from build123d import *

# Parameters (mm, degrees)
F0_W           = 31.75
F0_H           = 31.75
F1_DEPTH       = 38.1
F3_D           = 5.1054
F3_CBORE_D     = 8.73125
F3_CBORE_DEPTH = 25.4
F5_DEPTH       = 31.751
F7_D           = 4.0386
F7_DEPTH       = 9.49325
F7_TIP         = 1.213317848


with BuildPart() as f1:
    # F0 (on Top) → F1 (new body)
    with BuildSketch(Plane.XY):
        Rectangle(F0_W, F0_H)
    extrude(amount=F1_DEPTH)

    # F3 (through all)
    with Locations(Plane(origin=(0, 0, 0), x_dir=(1, 0, 0), z_dir=(0, 0, -1))):
        with Locations((0, 0)):
            CounterBoreHole(F3_D / 2, F3_CBORE_D / 2, F3_CBORE_DEPTH)

    # F4 (on face) → F5 (cut, through all)
    with BuildSketch(Plane.XZ.offset(15.875)):
        Polygon((34.4816722517, 22.1809802753), (33.3208667558, 31.6349823697), (8.1101945041, 28.5395010472), (9.271, 19.0854989528), align=None)
    extrude(amount=-F5_DEPTH, mode=Mode.SUBTRACT)

    # F7
    with Locations(Plane.XY.offset(38.1)):
        with Locations((12.065, -9.525), (12.065, 9.525)):
            Hole(F7_D / 2, depth=F7_DEPTH)
            with Locations((0, 0, -(F7_DEPTH + F7_TIP / 2))):  # 118° drill point
                Cone(0, F7_D / 2, F7_TIP, mode=Mode.SUBTRACT)


solid = f1.part
The model under review builds one solid part; all positions refer to its coordinate system, in mm. A direction names the side the tool comes from. Round coordinates to 2 decimals unless told otherwise and drop trailing zeros. Write each loop counter-clockwise with the first axis right and the second up, starting at its lowest first coordinate (ties: lowest second). Pieces come first, ordered by that corner, then holes. Notation, with made-up numbers: M 39.5,68 L 86.5,68 A33 ccw 86.5,107 Z; hole C 21.5,29.5 d5. An arc over 180 degrees is marked long. Use a Markdown table: item, result. Add a question column.
Q1. Machinability: for faces 1 (the face through (12.527, -0.222, 19.485)), 2 (the face through (10.2, -10.3, 33.4)), 3 (the face through (-3.46, 2.66, 12.52)), which of the approach directions +Z, -Z, +X, -X, +Y, -Y give a long, thin tool a straight path to every point of the face, cutting with its end or side? Answer none if there is none.
Q2. The part is to be moulded in two halves that separate along Z. For faces 4 (the face through (8.682, -0.222, 23.879)), 5 (the face through (2, 2, 25.4)), 6 (the face through (0, 15.875, 19)), 7 (the face through (-4, 0, 38.1)), say which applies: pulls with the +Z half, pulls with the -Z half, needs draft (parallel to the pull), parting line crosses it, or undercut.
Q3. To check wall thickness, follow line 1 (Y direction, x = 0, z = 28) (3 decimals); line 2 (Z direction, x = 12.5, y = -2.5); line 3 (X direction, y = 1.5, z = 22.5) (3 decimals). State the ranges of each line that lie inside material, in increasing order.
Q4. Insertion check: pin 1 (4.5 mm diameter, centred on x = 0, y = 0, fed in from -Z); pin 2 (3 mm diameter, centred on y = 9.5, z = 24.5, fed in from +X); pin 3 (1 mm diameter, centred on y = -8.5, z = 27, fed in from +X); pin 4 (7 mm diameter, centred on x = 0, y = 0, fed in from -Z). Each pin has a flat end and moves straight along its axis. Give the tip position at first contact, or say it passes through.
Q5. We need section B-B, the plane x = 0. State the section outline as (y, z) points (3 decimals), plus the area to 3 significant figures.
Q6. We need section D-D, the plane z = 32.5. State the section outline as (x, y) points (3 decimals).
Q7. We need section C-C, the plane z = 4. State the section outline as (x, y) points (3 decimals).
Q8. We need section A-A, the plane y = 0. State the section outline as (x, z) points (1 decimal), plus the area to 3 significant figures.
Findings below:
| question | item | result |
|---|---|---|
| 1 | face 1 | +Y, -Y |
| 1 | face 2 | +Z |
| 1 | face 3 | -Z |
| 2 | face 4 | undercut |
| 2 | face 5 | pulls with the -Z half |
| 2 | face 6 | needs draft |
| 2 | face 7 | pulls with the +Z half |
| 3 | line 1 | y = -15.875 to -2.553, 2.553 to 15.875 |
| 3 | line 2 | z = 0 to 19.48, 29.08 to 38.1 |
| 3 | line 3 | x = -15.875 to -4.1, 4.1 to 8.852 |
| 4 | pin 1 | passes through |
| 4 | pin 2 | stops at x = 8.79 |
| 4 | pin 3 | stops at x = 8.36 |
| 4 | pin 4 | stops at z = 25.4 |
| 5 | outline | M -15.875,0 L -4.366,0 L -4.366,25.4 L -2.553,25.4 L -2.553,38.1 L -15.875,38.1 Z; M 2.553,25.4 L 4.366,25.4 L 4.366,0 L 15.875,0 L 15.875,38.1 L 2.553,38.1 Z |
| 5 | area | 923 mm² |
| 6 | outline | M -15.875,-15.875 L 15.875,-15.875 L 15.875,15.875 L -15.875,15.875 Z; hole C 0,0 d5.105; hole C 12.065,-9.525 d4.039; hole C 12.065,9.525 d4.039 |
| 7 | outline | M -15.875,-15.875 L 15.875,-15.875 L 15.875,15.875 L -15.875,15.875 Z; hole C 0,0 d8.731 |
| 8 | outline | M -15.9,0 L -4.4,0 L -4.4,25.4 L -2.6,25.4 L -2.6,38.1 L -15.9,38.1 Z; M 2.6,25.4 L 4.4,25.4 L 4.4,0 L 15.9,0 L 15.9,19.9 L 9.3,19.1 L 8.1,28.5 L 15.9,29.5 L 15.9,38.1 L 2.6,38.1 Z |
| 8 | area | 854 mm² |
